For this review, use the dimensioned drawing (mm, ordinates from the lowest corner) and the shaded views. A direction names the side the tool comes from. Coordinates: 2 decimals unless noted, no trailing zeros. Loops run counter-clockwise (first coordinate to the right, second up) from the corner with the lowest first, then second, coordinate; pieces in that order, holes last. Notation, with made-up numbers: M 58.5,68 L 111.5,68 A7 cw 111.5,75 Z; hole C 76,69.5 d7. An arc over 180 degrees is marked long. Write item = value, one per line.
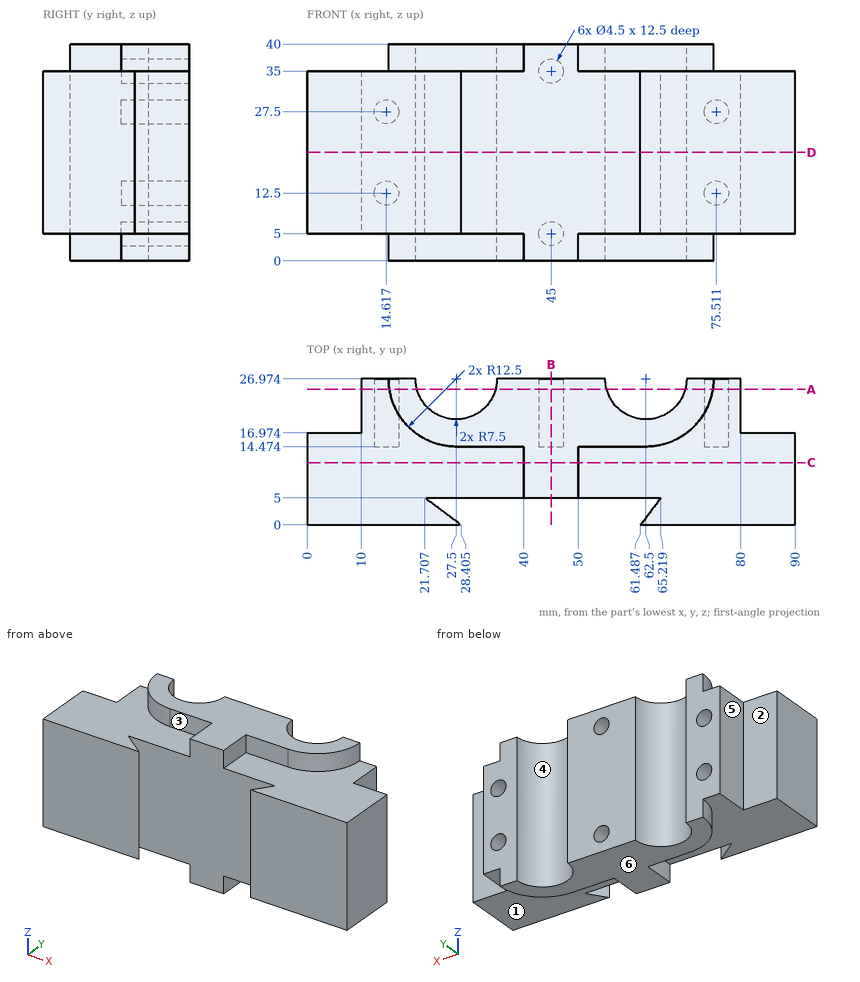
Q1. Add section D-D (z = 20). Write out the cut boundary in (x, y) (1 decimal).
Solved:
outline = M 0,0 L 28.4,0 L 21.7,5 L 65.2,5 L 61.5,0 L 90,0 L 90,17 L 80,17 L 80,27 L 70,27 A7.5 cw 55,27 L 35,27 A7.5 cw 20,27 L 10,27 L 10,17 L 0,17 Z
Q2. Add section A-A (y = 25). State how many separate pieces and enclosed holes the cut face has, and give its area (3 significant figures).
Solved:
separate_pieces = 3
enclosed_holes = 6
area = 1,440 mm²
Q3. For pin 1 Ø12 at (x, z) = (27.5, 6) entering from +Y (1 decimal); pin 2 Ø5 at (x, y) = (18, 7.5) entering from -Z; pin 3 Ø1 at (x, y) = (18, 16.5) entering from +Z, all flat-tipped, find the tip position at first contact; note any pin that passes through.
Solved:
pin_1 = 22.5
pin_2 = 5
pin_3 = 35
Q4. Add section B-B (x = 45). Write out the cut boundary in (y, z).
Solved:
outline = M 5,0 L 26.97,0 L 26.97,2.75 L 14.47,2.75 L 14.47,7.25 L 26.97,7.25 L 26.97,32.75 L 14.47,32.75 L 14.47,37.25 L 26.97,37.25 L 26.97,40 L 5,40 Z
Q5. Add section C-C (y = 11.5). Write out the cut boundary in (x, z), and give its area (3 significant figures).
Solved:
outline = M 0,5 L 40,5 L 40,0 L 50,0 L 50,5 L 90,5 L 90,35 L 50,35 L 50,40 L 40,40 L 40,35 L 0,35 Z
area = 2,800 mm²
Q6. Machinability: for the marked faces 1, 2 and 3, which of the approach directions +Z, -Z, +X, -X, +Y, -Y give a long, thin tool a straight path to every point of the face, cutting with its end or side? Answer none if there is none.
Solved:
face_1 = -Z, +X, -Y
face_2 = +Z, -Z, -X, +Y
face_3 = +Z, -X, -Y
Q7. For line 1 along Z through (x, y) = (45, 17.5); line 2 along X through (y, z) = (23, 8.5); line 3 along Y through (x, z) = (48, 29.5), list the stretches that pass through material, from the lowest coordinate up.
Solved:
line_1 = 0 to 2.75, 7.25 to 32.75, 37.25 to 40
line_2 = 10 to 21.14, 33.86 to 56.14, 68.86 to 80
line_3 = 5 to 26.97
Q8. Draft analysis for pull direction X (two halves, no side actions). For the marked faces 4, 5 and 6, state which applies: +X half, -X half, draft (parallel to the pull), parting line (faces both ways), or undercut.
Solved:
face_4 = undercut
face_5 = -X half
face_6 = draft
